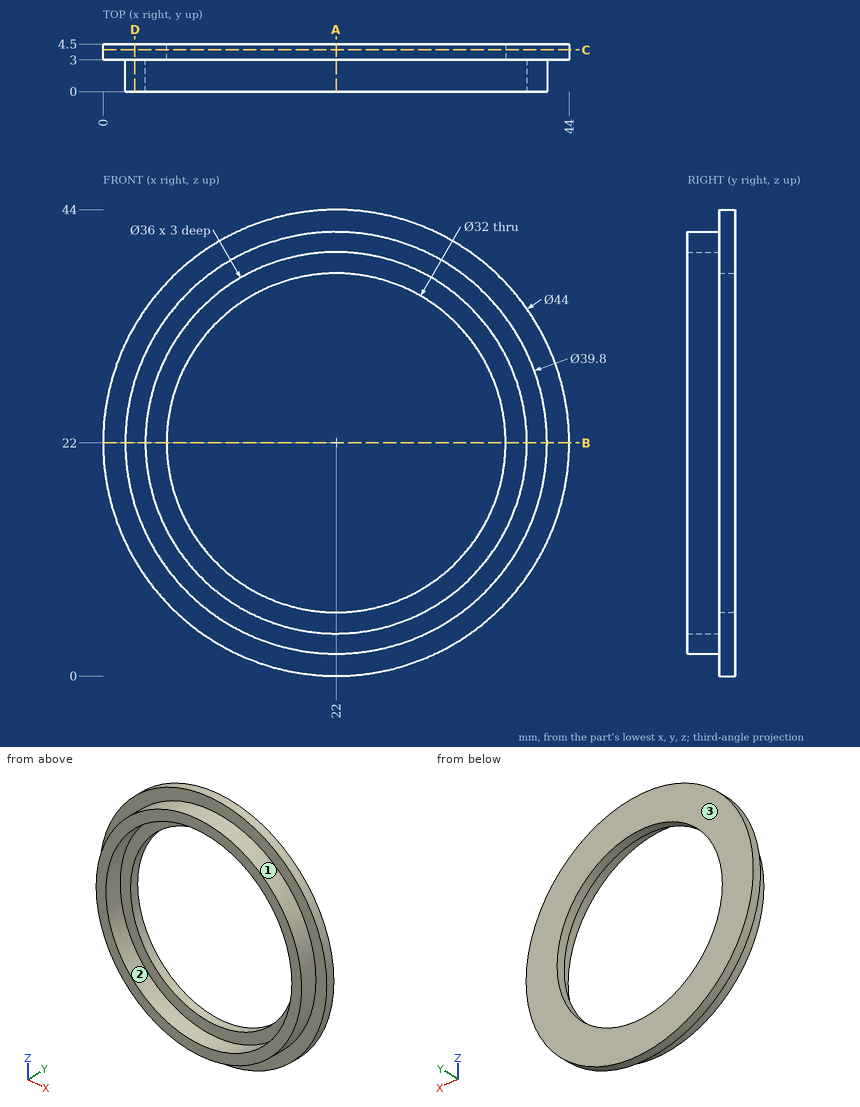
Geometry check sheet. Reference: drawing and pictorial views, mm from the part's lowest x, y, z. Give positions to 0.01 mm unless a question says otherwise; leave off trailing zeros. Write each loop counter-clockwise with the first axis right and the second up, starting at its lowest first coordinate (ties: lowest second). Pieces come first, ordered by that corner, then holes. Notation, with made-up numbers: M -10.75,17 L 1.25,17 A24 cw 1.25,41 Z; hole C 65.25,24 d11. An arc over 180 degrees is marked long. Use CSV: the item, a comma, the result in double quotes.
1) Release check for a two-part mould opening along X. For the marked faces 1, 2 and 3 record: released by +X, released by -X, zero draft, split by the parting line, or undercut.
Final values:
face 1,"split by the parting line"
face 2,"undercut"
face 3,"zero draft"
2) Cross-section at A-A (x = 22). Enter the section's corners in (y, z), plus the area to 3 significant figures.
Final values:
outline,"M 0,2.1 L 3,2.1 L 3,0 L 4.5,0 L 4.5,6 L 3,6 L 3,4 L 0,4 Z; M 0,40 L 3,40 L 3,38 L 4.5,38 L 4.5,44 L 3,44 L 3,41.9 L 0,41.9 Z"
area,"29.4 mm²"
3) Cross-section at D-D (x = 3). Enter the section's corners in (y, z).
Final values:
outline,"M 0,16.08 L 3,16.08 L 3,10.91 L 4.5,10.91 L 4.5,33.09 L 3,33.09 L 3,27.92 L 0,27.92 Z"
4) Material ranges on line 1 along Z through (x, y) = (22, 1.55); line 2 along Z through (x, y) = (22, 4.15); line 3 along X through (y, z) = (3.75, 14), recorded low to high.
Final values:
line 1,"2.1 to 4, 40 to 41.9"
line 2,"0 to 6, 38 to 44"
line 3,"1.51 to 8.14, 35.86 to 42.49"
5) Cross-section at C-C (y = 3.95). Enter the section's corners in (x, z), plus the area to 3 significant figures.
Final values:
outline,"C 22,22 d44; hole C 22,22 d32"
area,"716 mm²"
6) Go/stop test with flat-tipped pins: pin 1 Ø8 at (x, z) = (18.5, 13) entering from -Y; pin 2 Ø2 at (x, y) = (38, 1.5) entering from -Z. Record where each tip stops, or that it passes through.
Final values:
pin 1,"through"
pin 2,"z = 8.92"
7) Cross-section at B-B (z = 22). Enter the section's corners in (x, y), plus the area to 3 significant figures.
Final values:
outline,"M 0,3 L 2.1,3 L 2.1,0 L 4,0 L 4,3 L 6,3 L 6,4.5 L 0,4.5 Z; M 38,3 L 40,3 L 40,0 L 41.9,0 L 41.9,3 L 44,3 L 44,4.5 L 38,4.5 Z"
area,"29.4 mm²"
